For this review, take the finished solid that the model builds, in its own axes (mm). Face numbers are marked on the shaded views. A direction names the side the tool comes from. Round coordinates to 2 decimals unless told otherwise and drop trailing zeros. Write each loop counter-clockwise with the first axis right and the second up, starting at its lowest first coordinate (ties: lowest second). Pieces come first, ordered by that corner, then holes. Notation, with made-up numbers: M 3.5,3 L 45.5,3 A15 ccw 45.5,17 Z; hole C -11,63 d11. An arc over 180 degrees is marked long. Answer in a Markdown table with one row per item.
```python
from build123d import *

# Parameters (mm, degrees)
F0_W     = 93.749092
F0_H     = 90.747274
F1_DEPTH = 50.8
F2_R     = 19.189435
F3_DEPTH = 50.8
F5_DEPTH = 67.564


with BuildPart() as f1:
    # F0 (on Top) → F1 (new body)
    with BuildSketch(Plane.XY):
        Rectangle(F0_W, F0_H)
    extrude(amount=F1_DEPTH)

    # F2 (on face) → F3 (join)
    with BuildSketch(Plane.XY.offset(50.8)):
        Circle(F2_R)
    extrude(amount=F3_DEPTH)

    # F4 (on Front) → F5 (cut, symmetric)
    with BuildSketch(Plane.XZ):
        Polygon((59.805457, 108.200155), (-43.911207, 108.200155), (59.805457, 61.056212), align=None)
    extrude(amount=F5_DEPTH, both=True, mode=Mode.SUBTRACT)


solid = f1.part
```
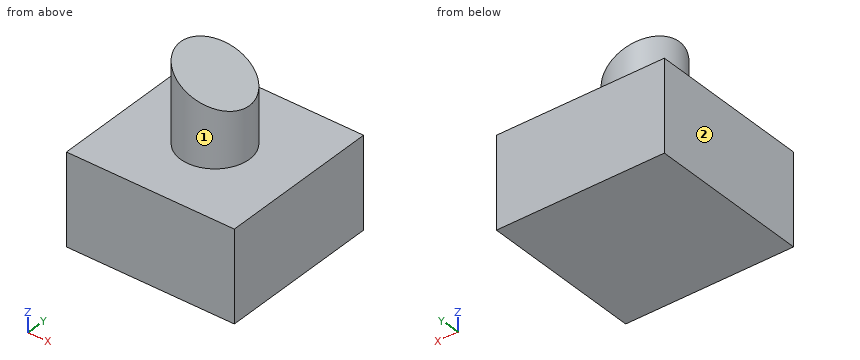
Q1. Machinability: for the marked faces 1 and 2, which of the approach directions +Z, -Z, +X, -X, +Y, -Y give a long, thin tool a straight path to every point of the face, cutting with its end or side? Answer none if there is none.
Found:
| item | result |
|---|---|
| face 1 | +Z |
| face 2 | +Z, -Z, -X, +Y, -Y |
Q2. Take a section at D-D (y = 21). State the section outline as (x, z) points.
Found:
| item | result |
|---|---|
| outline | M -46.87,0 L 46.87,0 L 46.87,50.8 L -46.87,50.8 Z |
Q3. Insertion check: P1, Ø3, axis at x = -30, y = -21.5, coming from the +Z side; P2, Ø5, axis at x = 1, y = -3.5, coming from the +Z side. Each pin has a flat end and moves straight along its axis. Give the tip position at first contact, or say it passes through.
Found:
| item | result |
|---|---|
| P1 | z = 50.8 |
| P2 | z = 88.92 |
Q4. For probe 1 along Z at (x, y) = (19, -41); probe 2 along X at (y, z) = (-6, 55); probe 3 along Z at (x, y) = (5.5, 7.5), list the stretches that pass through material, from the lowest coordinate up.
Found:
| item | result |
|---|---|
| probe 1 | 0 to 50.8 |
| probe 2 | -18.23 to 18.23 |
| probe 3 | 0 to 85.74 |
Q5. Take a section at A-A (y = 0). State the section outline as (x, z) points, then the cut area to 3 significant figures.
Found:
| item | result |
|---|---|
| outline | M -46.87,0 L 46.87,0 L 46.87,50.8 L 19.19,50.8 L 19.19,79.52 L -19.19,96.96 L -19.19,50.8 L -46.87,50.8 Z |
| area | 6,200 mm² |
Q6. Take a section at B-B (x = 40.5). State the section outline as (y, z) points.
Found:
| item | result |
|---|---|
| outline | M -45.37,0 L 45.37,0 L 45.37,50.8 L -45.37,50.8 Z |
Q7. Take a section at C-C (y = -15.5). State the section outline as (x, z) points, then the cut area to 3 significant figures.
Found:
| item | result |
|---|---|
| outline | M -46.87,0 L 46.87,0 L 46.87,50.8 L 11.31,50.8 L 11.31,83.1 L -11.31,93.38 L -11.31,50.8 L -46.87,50.8 Z |
| area | 5,610 mm² |
